from build123d import *

# Parameters (mm, degrees)
SKETCH1_W           = 6
SKETCH1_H           = 5
BOSS_EXTRUDE1_DEPTH = 11.5
SKETCH2_R           = 2.5
SKETCH2_R_2         = 1.8
BOSS_EXTRUDE2_DEPTH = 2.5
SKETCH3_R           = 1.8
CUT_EXTRUDE1_DEPTH  = 10
SKETCH4_W           = 0.75
SKETCH4_H           = 1.2
BOSS_EXTRUDE3_DEPTH = 0.3
SKETCH5_R           = 0.75
BOSS_EXTRUDE4_DEPTH = 0.6


with BuildPart() as part:
    # Sketch1 → Boss-Extrude1 (new body)
    with BuildSketch(Plane.XY):
        Rectangle(SKETCH1_W, SKETCH1_H)
    extrude(amount=BOSS_EXTRUDE1_DEPTH)

    # Sketch2 → Boss-Extrude2 (add)
    with BuildSketch(Plane.XY.offset(11.5)):
        Circle(SKETCH2_R)
        Circle(SKETCH2_R_2, mode=Mode.SUBTRACT)
    extrude(amount=BOSS_EXTRUDE2_DEPTH)

    # Sketch3 → Cut-Extrude1 (cut)
    with BuildSketch(Plane.XY.offset(11.5)):
        Circle(SKETCH3_R)
    extrude(amount=-CUT_EXTRUDE1_DEPTH, mode=Mode.SUBTRACT)

    # Sketch4 → Boss-Extrude3 (add)
    with BuildSketch(Plane.XZ.offset(2.5)):
        with Locations((3.375, 9.7)):
            Rectangle(SKETCH4_W, SKETCH4_H)
        with Locations((3.375, 6.5)):
            Rectangle(SKETCH4_W, SKETCH4_H)
        with Locations((3.375, 3)):
            Rectangle(SKETCH4_W, SKETCH4_H)
        with Locations((-3.375, 3)):
            Rectangle(SKETCH4_W, SKETCH4_H)
        with Locations((-3.375, 6.5)):
            Rectangle(SKETCH4_W, SKETCH4_H)
        with Locations((-3.375, 9.7)):
            Rectangle(SKETCH4_W, SKETCH4_H)
    extrude(amount=-BOSS_EXTRUDE3_DEPTH)

    # Sketch5 → Boss-Extrude4 (add)
    with BuildSketch(Plane.XZ.offset(2.5)):
        with Locations((0, 9)):
            Circle(SKETCH5_R)
        with Locations((0, 3)):
            Circle(SKETCH5_R)
    extrude(amount=BOSS_EXTRUDE4_DEPTH)


solid = part.part
For this review, take the finished solid that the model builds, in its own axes (mm). A direction names the side the tool comes from. Round coordinates to 2 decimals unless told otherwise and drop trailing zeros. Write each loop counter-clockwise with the first axis right and the second up, starting at its lowest first coordinate (ties: lowest second). Pieces come first, ordered by that corner, then holes. Notation, with made-up numbers: (-29.5, 4.25) -> (-8.5, 4.25) arc R31 ccw to (-8.5, 38.25) -> close; hole circle Ø6 at (61.5, 2). An arc over 180 degrees is marked (long way). Use CSV: the item, a comma, the result in double quotes.
(1) Consider section A-A, the plane z = 10. Give the boundary of the cut face in (x, y), plus the area to 3 significant figures.
Computed values:
outline,"(-3.75, -2.5) -> (3.75, -2.5) -> (3.75, -2.2) -> (3, -2.2) -> (3, 2.5) -> (-3, 2.5) -> (-3, -2.2) -> (-3.75, -2.2) -> close; hole circle Ø3.6 at (0, 0)"
area,"20.3 mm²"
(2) To check wall thickness, follow L1, parallel to Z at x = 3.25, y = -2.3; L2, parallel to Y at x = 0, z = 7.75; L3, parallel to Y at x = 0, z = 9.25. State the ranges of each line that lie inside material, in increasing order. Write a range as [from, to].
Computed values:
L1,"[2.4, 3.6], [5.9, 7.1], [9.1, 10.3]"
L2,"[-2.5, -1.8], [1.8, 2.5]"
L3,"[-3.1, -1.8], [1.8, 2.5]"
(3) For faces 5 (the face through (-0.098, -2.796, 9.744)), 6 (the face through (-1, 2, 14)), 7 (the face through (2.7, -0.2, 11.5)), 8 (the face through (0, 0, 0)), 9 (the face through (-0.54, -2.44, 12.73)), list the 3-axis set-ups (+Z, -Z, +X, -X, +Y, -Y) from which the entire face can be reached by the end or side of a thin tool; tool diameter is ignored.
Computed values:
face 5,"-Y"
face 6,"+Z, +X, -X, +Y, -Y"
face 7,"+Z, +X"
face 8,"-Z, +X, -X, +Y, -Y"
face 9,"+Z"
(4) Consider section D-D, the plane z = 3. Give the boundary of the cut face in (x, y).
Computed values:
outline,"(-3.75, -2.5) -> (-0.75, -2.5) -> (-0.75, -3.1) -> (0.75, -3.1) -> (0.75, -2.5) -> (3.75, -2.5) -> (3.75, -2.2) -> (3, -2.2) -> (3, 2.5) -> (-3, 2.5) -> (-3, -2.2) -> (-3.75, -2.2) -> close; hole circle Ø3.6 at (0, 0)"
(5) Draft analysis for pull direction X (two halves, no side actions). For faces 1 (the face through (0, 0, 1.5)), 2 (the face through (-0.163, -2.796, 2.268)), 3 (the face through (1.717, 0.541, 7.662)), 4 (the face through (-2.7, 0.2, 11.5)), state which applies: +X half, -X half, draft (parallel to the pull), parting line (faces both ways), or undercut.
Computed values:
face 1,"undercut"
face 2,"parting line"
face 3,"undercut"
face 4,"draft"
(6) Clearance check with flat-ended pins moving along their axes: P1, Ø2, axis at y = 2, z = 1.5, coming from the +X side; P2, Ø1.8, axis at x = 0, y = 1, coming from the +Z side; P3, Ø0.8, axis at x = -3.5, z = 10, coming from the +Y side; P4, Ø2, axis at x = 0, z = 5.5, coming from the -Y side. State where each tip first meets the part, or that it passes through.
Computed values:
P1,"x = 3"
P2,"z = 14"
P3,"y = -2.2"
P4,"y = -2.5"
(7) Consider section C-C, the plane x = 2.75. Give the boundary of the cut face in (y, z), plus the area to 3 significant figures.
Computed values:
outline,"(-2.5, 0) -> (2.5, 0) -> (2.5, 11.5) -> (-2.5, 11.5) -> close"
area,"57.5 mm²"
(8) Consider section B-B, the plane y = 0. Give the boundary of the cut face in (x, z), plus the area to 3 significant figures.
Computed values:
outline,"(-3, 0) -> (3, 0) -> (3, 11.5) -> (2.5, 11.5) -> (2.5, 14) -> (1.8, 14) -> (1.8, 1.5) -> (-1.8, 1.5) -> (-1.8, 14) -> (-2.5, 14) -> (-2.5, 11.5) -> (-3, 11.5) -> close"
area,"36.5 mm²"
